from build123d import *

# Parameters (mm, degrees)
BOX003_W          = 12
BOX003_H          = 9
BOX003_DEPTH      = 9
CYLINDER002_R     = 4.5
CYLINDER002_DEPTH = 12
CYLINDER003_R     = 4.5
CYLINDER003_DEPTH = 12
BOX002_W          = 5
BOX002_H          = 14
BOX002_DEPTH      = 11
BOX_W             = 15.2
BOX_H             = 68.2
BOX_DEPTH         = 18
BOX001_W          = 17
BOX001_H          = 70
BOX001_DEPTH      = 14
CHAMFER_SIZE      = 0.7
CHAMFER001_SIZE   = 0.7
CHAMFER005_SIZE   = 0.3


with BuildPart() as cubo002:
    # Box003 → Box003 (new body)
    with BuildSketch(Plane(origin=(-8, 8, -2), x_dir=(1, 0, 0), z_dir=(0, 0, 1))):
        with Locations((6, 4.5)):
            Rectangle(BOX003_W, BOX003_H)
    extrude(amount=BOX003_DEPTH)


with BuildPart() as cilindro001:
    # Cylinder002 → Cylinder002 (new body)
    with BuildSketch(Plane(origin=(-8, 8, 2.5), x_dir=(0, 0, -1), z_dir=(1, 0, 0))):
        Circle(CYLINDER002_R)
    extrude(amount=CYLINDER002_DEPTH)


with BuildPart() as fusion:
    # Cylinder003 → Cylinder003 (new body)
    with BuildSketch(Plane(origin=(-8, 17, 2.5), x_dir=(0, 0, -1), z_dir=(1, 0, 0))):
        Circle(CYLINDER003_R)
    extrude(amount=CYLINDER003_DEPTH)

    # Fusion: union Cilindro001
    add(cilindro001.part)


with BuildPart() as cubo001:
    # Box002 → Box002 (new body)
    with BuildSketch(Plane(origin=(1, 26, 2), x_dir=(1, 0, 0), z_dir=(0, 0, 1))):
        with Locations((2.5, 7)):
            Rectangle(BOX002_W, BOX002_H)
    extrude(amount=BOX002_DEPTH)


with BuildPart() as foroslot:
    # Box → Box (new body)
    with BuildSketch(Plane(origin=(-0.1, -0.1, -9), x_dir=(1, 0, 0), z_dir=(0, 0, 1))):
        with Locations((7.6, 34.1)):
            Rectangle(BOX_W, BOX_H)
    extrude(amount=BOX_DEPTH)


with BuildPart() as chamfer005:
    # Box001 → Box001 (new body)
    with BuildSketch(Plane(origin=(-1, -1, -4), x_dir=(1, 0, 0), z_dir=(0, 0, 1))):
        with Locations((8.5, 35)):
            Rectangle(BOX001_W, BOX001_H)
    extrude(amount=BOX001_DEPTH)

    # Cut: cut foroSlot
    add(foroslot.part, mode=Mode.SUBTRACT)

    # Cut001: cut Cubo001
    add(cubo001.part, mode=Mode.SUBTRACT)

    # Chamfer
    chamfer_edges = [chamfer005.edges().sort_by_distance(p)[0] for p in [
        (3.5, 26, 10),
        (6, 33, 10),
        (3.5, 40, 10),
        (1, 33, 10),
    ]]
    chamfer(chamfer_edges, length=CHAMFER_SIZE)

    # Chamfer001
    chamfer001_edges = [chamfer005.edges().sort_by_distance(p)[0] for p in [
        (-1, 34, 10),
        (7.5, -1, 10),
        (16, 34, 10),
        (7.5, 69, 10),
    ]]
    chamfer(chamfer001_edges, length=CHAMFER001_SIZE)

    # Cut002: cut Fusion
    add(fusion.part, mode=Mode.SUBTRACT)

    # Cut005: cut Cubo002
    add(cubo002.part, mode=Mode.SUBTRACT)

    # Chamfer005
    chamfer005_edges = [chamfer005.edges().sort_by_distance(p)[0] for p in [
        (7.5, -1, -4),
    ]]
    chamfer(chamfer005_edges, length=CHAMFER005_SIZE)


solid = chamfer005.part
Can you work these out from the model? Positions are in its coordinate system, mm. A direction names the side the tool comes from. Coordinates: 2 decimals unless noted, no trailing zeros. Loops run counter-clockwise (first coordinate to the right, second up) from the corner with the lowest first, then second, coordinate; pieces in that order, holes last. Notation, with made-up numbers: M 22,-12.5 L 76,-12.5 A26 cw 76,15.5 Z; hole C 5,29 d2. An arc over 180 degrees is marked long. Return JSON: item names as keys, results as strings. Group by question number.
Item 1: On a 3-axis mill with a long thin cutter (end or side, diameter ignored), from which of +Z, -Z, +X, -X, +Y, -Y can I reach the whole of each face in a straight line? I mean faces 4 (the cylindrical face through (-0.6, 21.5, 2.4)), 5 (the flat face through (7, -0.1, 2)), 6 (the flat face through (16, 34, 3)). Say none if no direction works.
Item 2: Imagine slicing it at C-C (y = 29.5). Please give me the cut outline in (x, z).
Item 3: I'm going to push flat-ended pins straight in: pin 1 Ø0.7 at (x, y) = (-1, 14) entering from +Z; pin 2 Ø2 at (x, y) = (5.5, 61) entering from -Z. Where does each tip first touch, or does it pass through?
Item 4: Imagine slicing it at B-B (z = 8.25). Please give me the cut outline in (x, y), and give its area (3 significant figures).
Item 5: Imagine slicing it at D-D (x = 8.5). Please give me the cut outline in (y, z).
Item 6: Imagine slicing it at A-A (x = 4.5). Please give me the cut outline in (y, z), and give its area (3 significant figures).
Item 7: Thinking about a two-plate mould opening in Z: for faces 1 (the flat face through (7, 68.1, 2)), 2 (the flat face through (7, 34, 9)), 3 (the cylindrical face through (-0.6, 3.5, 2.6)), which applies, released by +Z, released by -Z, zero draft, split by the parting line, or undercut?
Item 8: If I drill on L1, parallel to Y at x = 14, z = 6.75; L2, parallel to X at y = 56, z = 4.25; L3, parallel to Z at x = 6.75, y = 7.5, over which ranges is the centre line in solid material (lowest first)? Write a range as from..to.
Verdict:
{
 "1": {"face 4": "-X", "face 5": "-Z", "face 6": "+Z, -Z, +X, +Y, -Y"},
 "2": {"outline": "M -1,-4 L -0.1,-4 L -0.1,9 L 1,9 L 1,9.3 L 0.3,10 L -0.3,10 L -1,9.3 Z; M 6,9 L 15.1,9 L 15.1,-4 L 16,-4 L 16,9.3 L 15.3,10 L 6.7,10 L 6,9.3 Z"},
 "3": {"pin 1": "stops at z = 9.65", "pin 2": "stops at z = 9"},
 "4": {"outline": "M -1,-1 L 16,-1 L 16,69 L -1,69 Z; hole M -0.1,-0.1 L 15.1,-0.1 L 15.1,68.1 L -0.1,68.1 Z", "area": "153 mm^2"},
 "5": {"outline": "M -1,-3.7 L -0.7,-4 L -0.1,-4 L -0.1,9 L 68.1,9 L 68.1,-4 L 69,-4 L 69,9.3 L 68.3,10 L -0.3,10 L -1,9.3 Z"},
 "6": {"outline": "M -1,-3.7 L -0.7,-4 L -0.1,-4 L -0.1,9 L 26,9 L 26,9.3 L 25.3,10 L -0.3,10 L -1,9.3 Z; M 40,9 L 68.1,9 L 68.1,-4 L 69,-4 L 69,9.3 L 68.3,10 L 40.7,10 L 40,9.3 Z", "area": "78.4 mm^2"},
 "7": {"face 1": "zero draft", "face 2": "released by -Z", "face 3": "undercut"},
 "8": {"L1": "y = -1..-0.1, 68.1..69", "L2": "x = -1..-0.1, 15.1..16", "L3": "z = 9..10"}
}
